Geometry check sheet. Reference: the model listing, model coordinates, mm. A direction names the side the tool comes from. Round coordinates to 2 decimals unless told otherwise and drop trailing zeros. Write each loop counter-clockwise with the first axis right and the second up, starting at its lowest first coordinate (ties: lowest second). Pieces come first, ordered by that corner, then holes. Notation, with made-up numbers: (-27, 32.5) -> (10, 32.5) arc R33 ccw to (10, 67.5) -> close; hole circle Ø10 at (11, 38). An arc over 180 degrees is marked (long way). Put each result on its own line as item: value. Start each with the question number.
from build123d import *

# Parameters (mm, degrees)
SKETCH2_R               = 22.5
SKETCH2_R_2             = 2.25
BOSS_EXTRUDE1_DEPTH     = 3.175
SKETCH1_W               = 25.4
SKETCH1_H               = 35
SKETCH1_R               = 1.63
BOSS_EXTRUDE2_DEPTH     = 3.175
BOSS_EXTRUDE6_DEPTH     = 3.175
TOP_CONNECTION_SKETCH_W = 35
TOP_CONNECTION_SKETCH_H = 3.175


with BuildPart() as part:
    # Sketch2 → Boss-Extrude1 (new body)
    with BuildSketch(Plane(origin=(0, 236.49, 0), x_dir=(1, 0, 0), z_dir=(0, 1, 0))):
        with Locations(Location((0, 0, 0), (0, 0, 270))):
            Circle(SKETCH2_R)
        with Locations(Location((9.25, 16.02146997, 0), (0, 0, 270))):
            Circle(SKETCH2_R_2, mode=Mode.SUBTRACT)
        with Locations(Location((18.5, 0, 0), (0, 0, 270))):
            Circle(SKETCH2_R_2, mode=Mode.SUBTRACT)
        with Locations(Location((9.25, -16.02146997, 0), (0, 0, 270))):
            Circle(SKETCH2_R_2, mode=Mode.SUBTRACT)
        with Locations(Location((-9.25, -16.02146997, 0), (0, 0, 270))):
            Circle(SKETCH2_R_2, mode=Mode.SUBTRACT)
        with Locations(Location((-18.5, 0, 0), (0, 0, 270))):
            Circle(SKETCH2_R_2, mode=Mode.SUBTRACT)
        with Locations(Location((-9.25, 16.02146997, 0), (0, 0, 270))):
            Circle(SKETCH2_R_2, mode=Mode.SUBTRACT)
    extrude(amount=-BOSS_EXTRUDE1_DEPTH)

    # Sketch8 → Boss-Extrude6 (add)
    with BuildSketch(Plane(origin=(0, 236.49, 0), x_dir=(1, 0, 0), z_dir=(0, 1, 0))):
        Polygon((22.5, -17.648859957), (22.5, 0), (20.75, 0), (19.341522111, -11.495891545), (5.359057513, -21.852471315), align=None)
        Polygon((22.5, 0), (22.5, 17.648859957), (5.359057513, 21.852471315), (19.341522111, 11.495891545), (20.75, 0), align=None)
    extrude(amount=-BOSS_EXTRUDE6_DEPTH)



with BuildPart() as body_2:
    # Sketch1 → Boss-Extrude2 (new body)
    with BuildSketch(Plane(origin=(0, 0, 0), x_dir=(1, 0, 0), z_dir=(0, 1, 0))):
        with Locations((49.8, 0)):
            Rectangle(SKETCH1_W, SKETCH1_H)
        with Locations(Location((43.45, 0, 0), (0, 0, 270))):
            Circle(SKETCH1_R, mode=Mode.SUBTRACT)
        with Locations(Location((56.15, 0, 0), (0, 0, 270))):
            Circle(SKETCH1_R, mode=Mode.SUBTRACT)
        with Locations(Location((43.45, 12.7, 0), (0, 0, 270))):
            Circle(SKETCH1_R, mode=Mode.SUBTRACT)
        with Locations(Location((56.15, 12.7, 0), (0, 0, 270))):
            Circle(SKETCH1_R, mode=Mode.SUBTRACT)
        with Locations(Location((43.45, -12.7, 0), (0, 0, 270))):
            Circle(SKETCH1_R, mode=Mode.SUBTRACT)
        with Locations(Location((56.15, -12.7, 0), (0, 0, 270))):
            Circle(SKETCH1_R, mode=Mode.SUBTRACT)
    extrude(amount=BOSS_EXTRUDE2_DEPTH)


with BuildPart() as part_1:
    add(part.part)

    add(body_2.part)  # Sweep1 merges body 2
    # Sweep1: sweep along a curve in space
    with BuildLine() as sweep1_path:
        Line((22.5, 236.49, 0), (54.871837923, 219.215989902, 0))
        Line((70.25, 132.157447282, 0), (54.871837923, 219.215989902, 0))
        Line((62.5, 3.175, 0), (70.25, 132.157447282, 0))
    # Top_Connection_Sketch → Sweep1 (sweep)
    with BuildSketch(Plane(origin=(22.5, 0, 0), x_dir=(0, 0, -1), z_dir=(1, 0, 0))):
        with Locations((0, 234.9025)):
            Rectangle(TOP_CONNECTION_SKETCH_W, TOP_CONNECTION_SKETCH_H)
    sweep(path=sweep1_path.line, transition=Transition.RIGHT)


solid = part_1.part
(1) Set-up check for faces 1 (the flat face through (37.63, 225.24, 0.24)), 2 (the flat face through (0, 233.315, 0)), 3 (the flat face through (50, 0, 0)): record each of +Z, -Z, +X, -X, +Y, -Y from which the full face is reachable in a straight line by a thin tool's end or side.
(2) Sectioned sample at D-D (x = 50). Record the cut outline in (y, z) (3 decimals).
(3) Sectioned sample at C-C (y = 186). Record the cut outline in (x, z).
(4) Sectioned sample at A-A (x = 18.5). Record the cut outline in (y, z) (3 decimals), and give its area (3 significant figures).
(5) Mould release check, pull along Z, two halves, no side actions. Record for faces 4 (the cylindrical face through (11.147, 234.925, -14.812)), 5 (the cylindrical face through (11.15, 234.92, 17.23)), 6 (the flat face through (63.51, 66.68, 0.24)), 7 (the flat face through (68, 126, -17.5)): +Z half, -Z half, draft (parallel to the pull), parting line (faces both ways), or undercut.
(6) Sectioned sample at B-B (x = -9.25). Record the cut outline in (y, z) (3 decimals).
(7) Material ranges on L1, parallel to X at y = 1.75, z = 12.7; L2, parallel to Z at x = 43, y = 2; L3, parallel to Y at x = 3.5, z = -17 (3 decimals), recorded low to high. Write a range as from..to.
(8) Go/stop test with flat-tipped pins: pin 1 Ø3.5 at (y, z) = (2, 6.5) entering from -X; pin 2 Ø2 at (y, z) = (198.5, -12.5) entering from +X; pin 3 Ø1 at (y, z) = (129.5, 17.5) entering from -X. Record where each tip stops, or that it passes through.
Found:
1. face 1: +Z, -Z, -X
1. face 2: +Z, -Z, -X, -Y
1. face 3: +Z, -Z, +X, -X, -Y
2. outline: (0, -17.5) -> (3.175, -17.5) -> (3.175, 17.5) -> (0, 17.5) -> close; (218.641, -17.5) -> (221.816, -17.5) -> (221.816, 17.5) -> (218.641, 17.5) -> close
3. outline: (57.89, -17.5) -> (60.74, -17.5) -> (60.74, 17.5) -> (57.89, 17.5) -> close
4. outline: (233.315, -18.63) -> (236.49, -18.63) -> (236.49, -2.25) -> (233.315, -2.25) -> close; (233.315, 2.25) -> (236.49, 2.25) -> (236.49, 18.63) -> (233.315, 18.63) -> close
4. area: 104 mm2
5. face 4: undercut
5. face 5: undercut
5. face 6: draft
5. face 7: -Z half
6. outline: (233.315, -20.511) -> (236.49, -20.511) -> (236.49, -18.271) -> (233.315, -18.271) -> close; (233.315, -13.771) -> (236.49, -13.771) -> (236.49, 13.771) -> (233.315, 13.771) -> close; (233.315, 18.271) -> (236.49, 18.271) -> (236.49, 20.511) -> (233.315, 20.511) -> close
7. L1: 37.1..41.82, 45.08..54.52, 57.78..62.5
7. L2: -17.5..-14.27, -11.13..-1.57, 1.57..11.13, 14.27..17.5
7. L3: 233.315..236.49
8. pin 1: x = 37.1
8. pin 2: x = 58.71
8. pin 3: x = 67.25
